For this review, take the finished solid that the model builds, in its own axes (mm). Give positions to 0.01 mm unless a question says otherwise; leave off trailing zeros. Order: outer loops, then holes, each group sorted by start corner. A loop starts at its lowest first (then second) coordinate and runs counter-clockwise, first axis right, second up. Notation, with made-up numbers: (-24.5, 88.25) -> (3.5, 88.25) arc R24 ccw to (3.5, 125.25) -> close; hole circle Ø4 at (0.5, -4). An arc over 180 degrees is marked (long way). Return JSON: item names as keys, results as strings. Group by question number.
1) The part is to be moulded in two halves that separate along X. For faces 1 (the face through (-2.4, 16.2, -53.2)), 2 (the face through (1, 0, 15)), 3 (the face through (21.84, 15.78, 69.34)), 4 (the face through (-47.2, 16.2, 24.1)), say which applies: released by +X, released by -X, zero draft, split by the parting line, or undercut.
2) Add section C-C (y = 4). Give the boundary of the cut face in (x, z), then the cut area to 3 significant figures.
3) Add section A-A (z = 0). Give the boundary of the cut face in (x, y), then the cut area to 3 significant figures.
4) Insertion check: P1, Ø8, axis at y = 19, z = 19.5, coming from the +X side; P2, Ø10, axis at y = 15, z = 45, coming from the +X side; P3, Ø5, axis at y = 14.5, z = 29, coming from the +X side. Each pin has a flat end and moves straight along its axis. Give the tip position at first contact, or say it passes through.
5) Add section D-D (z = 60). Give the boundary of the cut face in (x, y), then the cut area to 3 significant figures.
6) Add section B-B (x = 45). Give the boundary of the cut face in (y, z), then the cut area to 3 significant figures.
7) To check wall thickness, follow line 1 along X through (y, z) = (10, 25); line 2 along X through (y, z) = (16, -50); line 3 along X through (y, z) = (18, 55). State the ranges of each line that lie inside material, in increasing order.
from build123d import *

# Parameters (mm, degrees)
SKETCH1_R           = 72.7
BOSS_EXTRUDE1_DEPTH = 32
SKETCH2_R           = 4
CUT_EXTRUDE1_DEPTH  = 108.678131485
CIRPATTERN1_COUNT   = 3
SKETCH3_R           = 1.5
CUT_EXTRUDE2_DEPTH  = 108.678131485
SKETCH4_R           = 4
CUT_EXTRUDE3_DEPTH  = 108.678131485


with BuildPart() as part:
    # Sketch1 → Boss-Extrude1 (new body)
    with BuildSketch(Plane(origin=(0, 0, 0), x_dir=(1, 0, 0), z_dir=(0, 1, 0))):
        with Locations(Location((0, 0, 0), (0, 0, 270))):
            Circle(SKETCH1_R)
    extrude(amount=BOSS_EXTRUDE1_DEPTH)

    # Sketch2 → Cut-Extrude1 (cut, through all)
    with BuildSketch(Plane(origin=(0, 32, 0), x_dir=(1, 0, 0), z_dir=(0, 1, 0))):
        with Locations(Location((0, 50, 0), (0, 0, 270))):
            Circle(SKETCH2_R)
    cut_extrude1 = extrude(amount=-CUT_EXTRUDE1_DEPTH, mode=Mode.SUBTRACT)

    # CirPattern1: Cut-Extrude1 ×3 about axis
    cirpattern1_axis = Axis((0, 0, 0), (0, 1, 0))
    for i in range(1, CIRPATTERN1_COUNT):
        add(cut_extrude1.rotate(cirpattern1_axis, i * 360 / CIRPATTERN1_COUNT), mode=Mode.SUBTRACT)

    # Sketch3 → Cut-Extrude2 (cut, through all)
    with BuildSketch(Plane(origin=(0, 32, 0), x_dir=(1, 0, 0), z_dir=(0, 1, 0))):
        with Locations(Location((0, -68, 0), (0, 0, 270))):
            Circle(SKETCH3_R)
    extrude(amount=-CUT_EXTRUDE2_DEPTH, mode=Mode.SUBTRACT)

    # Sketch4 → Cut-Extrude3 (cut, through all)
    with BuildSketch(Plane(origin=(0, 32, 0), x_dir=(1, 0, 0), z_dir=(0, 1, 0))):
        with Locations(Location((0, 0, 0), (0, 0, 270))):
            Circle(SKETCH4_R)
    extrude(amount=-CUT_EXTRUDE3_DEPTH, mode=Mode.SUBTRACT)


solid = part.part
Evaluation:
{
 "1": {"face 1": "undercut", "face 2": "zero draft", "face 3": "split by the parting line", "face 4": "undercut"},
 "2": {"outline": "circle Ø145.4 at (0, 0); hole circle Ø8 at (-43.3, 25); hole circle Ø8 at (0, -50); hole circle Ø8 at (0, 0); hole circle Ø3 at (0, 68); hole circle Ø8 at (43.3, 25)", "area": "16,400 mm^2"},
 "3": {"outline": "(-72.7, 0) -> (-4, 0) -> (-4, 32) -> (-72.7, 32) -> close; (4, 0) -> (72.7, 0) -> (72.7, 32) -> (4, 32) -> close", "area": "4,400 mm^2"},
 "4": {"P1": "x = 71.03", "P2": "x = 60.71", "P3": "x = 67.7"},
 "5": {"outline": "(-41.05, 0) -> (41.05, 0) -> (41.05, 32) -> (-41.05, 32) -> close", "area": "2,630 mm^2"},
 "6": {"outline": "(0, -57.1) -> (32, -57.1) -> (32, 21.38) -> (0, 21.38) -> close; (0, 28.62) -> (32, 28.62) -> (32, 57.1) -> (0, 57.1) -> close", "area": "3,420 mm^2"},
 "7": {"line 1": "-68.27 to -47.3, -39.3 to 39.3, 47.3 to 68.27", "line 2": "-52.78 to -4, 4 to 52.78", "line 3": "-47.54 to 47.54"}
}
